Part print with two shaded views. Sizes in mm from the minimum x, y, z corner. A direction names the side the tool comes from. Round coordinates to 2 decimals unless told otherwise and drop trailing zeros. Write each loop counter-clockwise with the first axis right and the second up, starting at its lowest first coordinate (ties: lowest second). Pieces come first, ordered by that corner, then holes. Notation, with made-up numbers: (17, -16.5) - (40, -16.5) arc R35 ccw to (40, 19.5) - close; hole circle Ø8 at (69.25, 22). An arc over 180 degrees is marked (long way). Answer as a JSON object with one key per item and string values. Group by question number.
Item 1: Flat gauge pins, fed straight in: pin 1 (8 mm diameter, centred on x = 39.5, y = 5.5, fed in from +Z); pin 2 (11.5 mm diameter, centred on x = 46, z = 17, fed in from -Y); pin 3 (3 mm diameter, centred on x = 46.5, z = 15.5, fed in from +Y); pin 4 (14 mm diameter, centred on x = 45, y = 9, fed in from +Z). Where does each tip first touch, or does it go through?
Item 2: Slice it at A-A, the plane z = 16.5. List the corners of the cut face in (x, y).
Item 3: Probe line 1 (X direction, y = 19.25, z = 26); line 2 (Z direction, x = 48, y = 18.25) (1 decimal); line 3 (Y direction, x = 42, z = 20). List the from-to ranges inside material, lowest first. Write a range as from..to.
Item 4: Slice it at C-C, the plane x = 40. List the corners of the cut face in (y, z) (1 decimal), then the cut area to 3 significant figures.
Item 5: Slice it at D-D, the plane y = 23.75. List the corners of the cut face in (x, z), then the cut area to 3 significant figures.
Item 6: Slice it at B-B, the plane y = 12.5. List the corners of the cut face in (x, z) (1 decimal).
Item 7: Which spindle directions (+Z, -Z, +X, -X, +Y, -Y) get a long thin tool onto all of the face, cutting with end or side? Do the marked faces 1, 2, 3, 4 and 5. Say none if no direction does.
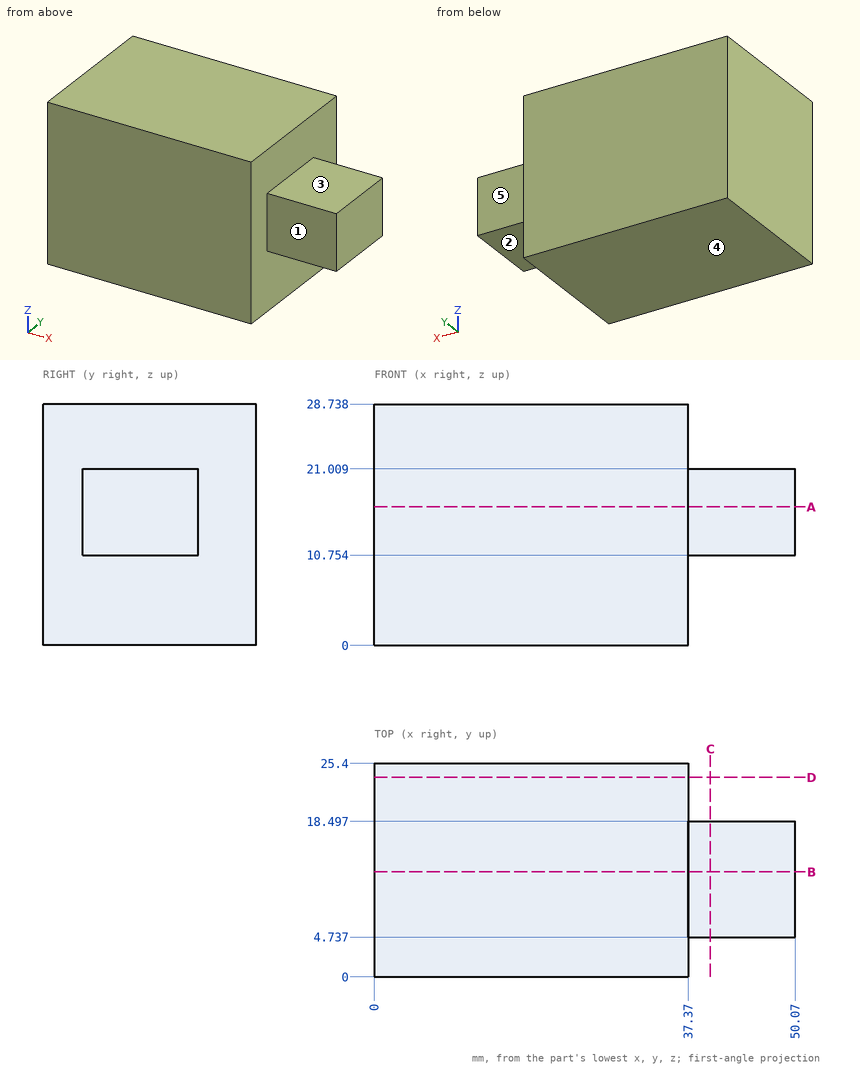
Geometry says:
{
 "1": {"pin 1": "stops at z = 28.74", "pin 2": "stops at y = 4.74", "pin 3": "stops at y = 18.5", "pin 4": "stops at z = 21.01"},
 "2": {"outline": "(0, 0) - (37.37, 0) - (37.37, 4.74) - (50.07, 4.74) - (50.07, 18.5) - (37.37, 18.5) - (37.37, 25.4) - (0, 25.4) - close"},
 "3": {"line 1": "x = 0..37.37", "line 2": "z = 10.8..21", "line 3": "y = 4.74..18.5"},
 "4": {"outline": "(4.7, 10.8) - (18.5, 10.8) - (18.5, 21) - (4.7, 21) - close", "area": "141 mm^2"},
 "5": {"outline": "(0, 0) - (37.37, 0) - (37.37, 28.74) - (0, 28.74) - close", "area": "1,070 mm^2"},
 "6": {"outline": "(0, 0) - (37.4, 0) - (37.4, 10.8) - (50.1, 10.8) - (50.1, 21) - (37.4, 21) - (37.4, 28.7) - (0, 28.7) - close"},
 "7": {"face 1": "+Z, -Z, +X, -Y", "face 2": "-Z, +X, +Y, -Y", "face 3": "+Z, +X, +Y, -Y", "face 4": "-Z, +X, -X, +Y, -Y", "face 5": "+Z, -Z, +X, +Y"}
}
